Read the model definition and answer for the solid it produces. Units are mm, in the model's axes. Face numbers are marked on the shaded views. A direction names the side the tool comes from. Round coordinates to 2 decimals unless told otherwise and drop trailing zeros. Write each loop counter-clockwise with the first axis right and the second up, starting at its lowest first coordinate (ties: lowest second). Pieces come first, ordered by that corner, then holes. Notation, with made-up numbers: (72.25, 70) - (90.25, 70) arc R23 cw to (90.25, 81) - close; hole circle Ø5 at (86.5, 54). An arc over 180 degrees is marked (long way). Answer as CSV lines item,"result". Start each with the question number.
1) Which of the six approach directions +Z, -Z, +X, -X, +Y, -Y give full straight-line access (tool end or side, diameter ignored) to the marked faces 4, 5, 6 and 7?
2) Find section C-C on x = -3.75. Determine the outline of the cut face in (y, z), then the cut area to 3 significant figures.
3) Consider line 1 along Y through (x, z) = (-3.75, 18.5); line 2 along X through (y, z) = (-2.35, 46); line 3 along Z through (x, y) = (-5, -3.85). Determine where each line is inside the solid, lowest interval first.
4) Find section B-B on z = 20.5. Determine the outline of the cut face in (x, y).
5) Find section D-D on y = -2.5. Determine the outline of the cut face in (x, z), then the cut area to 3 significant figures.
6) For a pull along Y with two mould halves and no side action, classify the marked faces 1, 2 and 3 as +Y half, -Y half, draft (parallel to the pull), parting line (faces both ways), or undercut.
7) Find section A-A on y = 5. Determine the outline of the cut face in (x, z).
8) Each of these flat-tipped pins is pushed along its axis until it touches: pin 1 (0.8 mm diameter, centred on x = -7.5, y = 7.5, fed in from -Z); pin 2 (1.5 mm diameter, centred on x = -3, y = -3, fed in from -Z); pin 3 (2 mm diameter, centred on x = -6.5, z = 14, fed in from -Y). Where does it stop, or does it pass through?
from build123d import *

# Parameters (mm, degrees)
SKETCH1_W           = 10
SKETCH1_H           = 10
SKETCH1_W_2         = 7
SKETCH1_H_2         = 7
BOSS_EXTRUDE1_DEPTH = 50
SKETCH2_W           = 7
SKETCH2_H           = 7
BOSS_EXTRUDE2_DEPTH = 5
SKETCH3_R           = 4
CUT_EXTRUDE1_DEPTH  = 5
SKETCH4_R           = 2.5
SKETCH4_R_2         = 0.5
BOSS_EXTRUDE3_DEPTH = 5
SKETCH5_R           = 4.75
SKETCH5_R_2         = 3.25
BOSS_EXTRUDE4_DEPTH = 10


with BuildPart() as part:
    # Sketch1 → Boss-Extrude1 (new body)
    with BuildSketch(Plane.XY):
        with Locations((-5, 5)):
            Rectangle(SKETCH1_W, SKETCH1_H)
        with Locations((-5, 5)):
            Rectangle(SKETCH1_W_2, SKETCH1_H_2, mode=Mode.SUBTRACT)
    extrude(amount=BOSS_EXTRUDE1_DEPTH)

    # Sketch2 → Boss-Extrude2 (add)
    with BuildSketch(Plane.XY.offset(50)):
        with Locations((-5, 5)):
            Rectangle(SKETCH2_W, SKETCH2_H)
    extrude(amount=-BOSS_EXTRUDE2_DEPTH)

    # Sketch3 → Cut-Extrude1 (cut)
    with BuildSketch(Plane.XY.offset(50)):
        with Locations((-5, 5)):
            Circle(SKETCH3_R)
    extrude(amount=-CUT_EXTRUDE1_DEPTH, mode=Mode.SUBTRACT)

    # Sketch4 → Boss-Extrude3 (add)
    with BuildSketch(Plane.XZ):
        with Locations(Location((-5, 46, 0), (0, 0, 180))):
            Circle(SKETCH4_R)
        with Locations((-5, 46)):
            Circle(SKETCH4_R_2, mode=Mode.SUBTRACT)
    extrude(amount=BOSS_EXTRUDE3_DEPTH)

    # Sketch5 → Boss-Extrude4 (add)
    with BuildSketch(Plane.XY.offset(50)):
        with Locations((-5, 5)):
            Circle(SKETCH5_R)
        with Locations((-5, 5)):
            Circle(SKETCH5_R_2, mode=Mode.SUBTRACT)
    extrude(amount=BOSS_EXTRUDE4_DEPTH)


solid = part.part
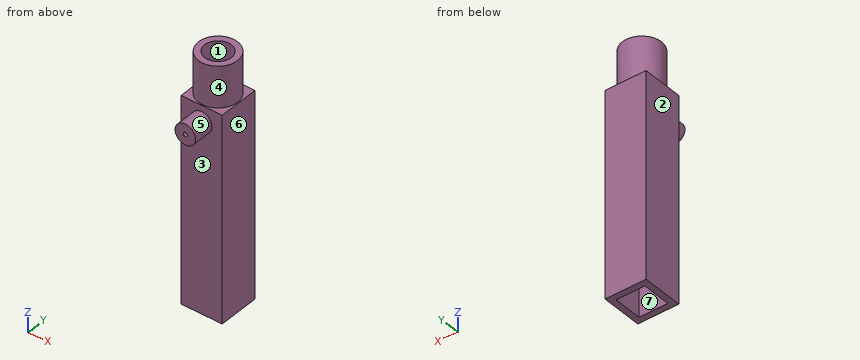
Check values:
1,face 4,"+Z"
1,face 5,"-Y"
1,face 6,"+Z, -Z, +X, +Y, -Y"
1,face 7,"-Z"
2,outline,"(-5, 43.83) - (0, 43.83) - (0, 0) - (1.5, 0) - (1.5, 45) - (1.2, 45) - (1.2, 50) - (2, 50) - (2, 60) - (0.42, 60) - (0.42, 50) - (0, 50) - (0, 48.17) - (-5, 48.17) - close; (8, 50) - (8.8, 50) - (8.8, 45) - (8.5, 45) - (8.5, 0) - (10, 0) - (10, 50) - (9.58, 50) - (9.58, 60) - (8, 60) - close"
2,area,"200 mm^2"
3,line 1,"y = 0 to 1.5, 8.5 to 10"
3,line 2,"x = -7.5 to -5.5, -4.5 to -2.5"
3,line 3,"z = 43.5 to 45.5, 46.5 to 48.5"
4,outline,"(-10, 0) - (0, 0) - (0, 10) - (-10, 10) - close; hole (-8.5, 1.5) - (-1.5, 1.5) - (-1.5, 8.5) - (-8.5, 8.5) - close"
5,outline,"circle Ø5 at (-5, 46); hole circle Ø1 at (-5, 46)"
5,area,"18.8 mm^2"
6,face 1,"undercut"
6,face 2,"draft"
6,face 3,"-Y half"
7,outline,"(-10, 0) - (-8.5, 0) - (-8.5, 45) - (-9, 45) - (-9, 50) - (-8.25, 50) - (-8.25, 60) - (-9.75, 60) - (-9.75, 50) - (-10, 50) - close; (-1.75, 50) - (-1, 50) - (-1, 45) - (-1.5, 45) - (-1.5, 0) - (0, 0) - (0, 50) - (-0.25, 50) - (-0.25, 60) - (-1.75, 60) - close"
8,pin 1,"stops at z = 50"
8,pin 2,"stops at z = 43.83"
8,pin 3,"stops at y = 0"
